Work out the finished part from the listing and answer in its coordinate system (mm). Face numbers are marked on the shaded views. A direction names the side the tool comes from. Coordinates: 2 decimals unless noted, no trailing zeros. Loops run counter-clockwise (first coordinate to the right, second up) from the corner with the lowest first, then second, coordinate; pieces in that order, holes last. Notation, with made-up numbers: (10.25, 87) - (64.25, 87) arc R24 cw to (64.25, 103) - close; hole circle Ø9 at (45, 13). An arc over 180 degrees is marked (long way). Write each question's results on one line, items separated by ' | '. Start each with the question number.
1. A cutting plane is placed at B-B on z = 0. Determine the outline of the cut face in (x, y), then the cut area to 3 significant figures.
2. Which of the six approach directions +Z, -Z, +X, -X, +Y, -Y give full straight-line access (tool end or side, diameter ignored) to the marked faces 5, 6, 7, 8 and 9?
3. Each of these flat-tipped pins is pushed along its axis until it touches: P1, Ø0.8, axis at x = 1, z = -18.5, coming from the -Y side; P2, Ø2.5, axis at x = -4, y = -10.5, coming from the -Z side; P3, Ø1.2, axis at x = -4.5, y = 1, coming from the +Z side. Where does it stop, or does it pass through?
4. A cutting plane is placed at C-C on z = -9.5. Determine the outline of the cut face in (x, y), then the cut area to 3 significant figures.
5. A cutting plane is placed at D-D on y = 2. Determine the outline of the cut face in (x, z), then the cut area to 3 significant figures.
6. Find the intervals of material crossed by line 1 along Z through (x, y) = (0, 3.4); line 2 along Y through (x, z) = (2.5, -9); line 3 along X through (y, z) = (-15.9, 0), in increasing order. Write a range as [from, to].
7. A cutting plane is placed at A-A on x = 0. Determine the outline of the cut face in (y, z), then the cut area to 3 significant figures.
8. Determine the mould class of the marked faces 1, 2, 3 and 4 for opening direction Z: released by +Z, released by -Z, zero draft, split by the parting line, or undercut.
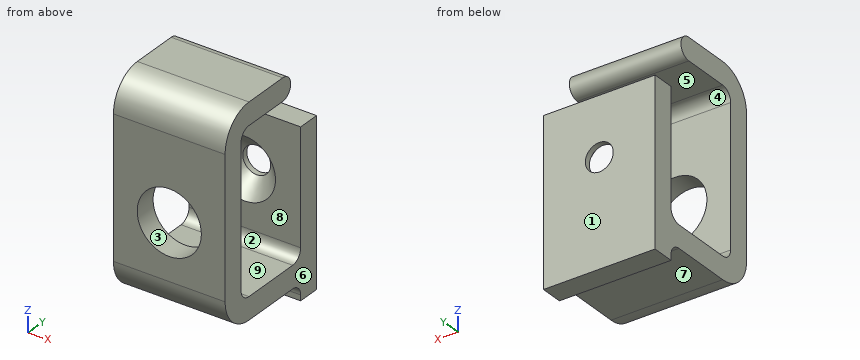
from build123d import *

# Parameters (mm, degrees)
PAD_DEPTH        = 10
HOLE_D           = 5
HOLE_CSINK_D     = 11
HOLE_CSINK_ANGLE = 90
SKETCH002_R      = 5.75
POCKET_DEPTH     = 19.001


with BuildPart() as part:
    # Sketch → Pad (new body, symmetric)
    with BuildSketch(Plane.YZ):
        with BuildLine():
            Line((0, -10), (0, 10.5))
            Line((0, 10.5), (4, 10.5))
            Line((4, 10.5), (4, -19))
            Line((4, -19), (0, -19))
            Line((0, -19), (0, -18))
            ThreePointArc((0, -18), (-0.585786, -16.585786), (-2, -16))
            Line((-2, -16), (-13, -16))
            ThreePointArc((-19, -10), (-17.242641, -14.242641), (-13, -16))
            Line((-19, -10), (-19, 15))
            ThreePointArc((-13, 21), (-17.242641, 19.242641), (-19, 15))
            Line((-13, 21), (-4.5, 21))
            ThreePointArc((-4.5, 17), (-2.5, 19), (-4.5, 21))
            Line((-13, 17), (-4.5, 17))
            ThreePointArc((-13, 17), (-14.414214, 16.414214), (-15, 15))
            Line((-15, -10), (-15, 15))
            ThreePointArc((-15, -10), (-14.414214, -11.414214), (-13, -12))
            Line((-2, -12), (-13, -12))
            ThreePointArc((-2, -12), (-0.585786, -11.414214), (0, -10))
        make_face()
    extrude(amount=PAD_DEPTH, both=True)

    # Hole (through all)
    with Locations(Plane.XZ):
        with Locations((0, 0)):
            CounterSinkHole(HOLE_D / 2, HOLE_CSINK_D / 2, counter_sink_angle=HOLE_CSINK_ANGLE)

    # Sketch002 → Pocket (cut, through all)
    with BuildSketch(Plane.XZ):
        Circle(SKETCH002_R)
    extrude(amount=POCKET_DEPTH, mode=Mode.SUBTRACT)


solid = part.part
Values:
1) outline: (-10, -19) - (-5.75, -19) - (-5.75, -15) - (-10, -15) - close; (-10, 0) - (-5.5, 0) - (-2.5, 3) - (-2.5, 4) - (-10, 4) - close; (2.5, 3) - (5.5, 0) - (10, 0) - (10, 4) - (2.5, 4) - close; (5.75, -19) - (10, -19) - (10, -15) - (5.75, -15) - close | area: 85.0 mm^2
2) face 5: +X, -X, +Y | face 6: +Z, -Z, +X, +Y, -Y | face 7: -Z, +X, -X, -Y | face 8: +Z, +X, -X | face 9: +X, -X
3) P1: y = 0 | P2: z = -16 | P3: z = 10.5
4) outline: (-10, -19) - (10, -19) - (10, -15) - (-10, -15) - close; (-10, 0) - (10, 0) - (10, 4) - (-10, 4) - close | area: 160 mm^2
5) outline: (-10, -19) - (10, -19) - (10, 10.5) - (-10, 10.5) - close; hole circle Ø7 at (0, 0) | area: 552 mm^2
6) line 1: [-19, -2.5], [2.5, 10.5] | line 2: [-19, -15], [0, 4] | line 3: [-10, -5.75], [5.75, 10]
7) outline: (-19, -10) arc R6 ccw to (-13, -16) - (-2, -16) arc R2 cw to (0, -18) - (0, -19) - (4, -19) - (4, -2.5) - (3, -2.5) - (0, -5.5) - (0, -10) arc R2 cw to (-2, -12) - (-13, -12) arc R2 cw to (-15, -10) - (-15, -5.75) - (-19, -5.75) - close; (-19, 5.75) - (-15, 5.75) - (-15, 15) arc R2 cw to (-13, 17) - (-4.5, 17) arc R2 ccw to (-4.5, 21) - (-13, 21) arc R6 ccw to (-19, 15) - close; (0, 5.5) - (3, 2.5) - (4, 2.5) - (4, 10.5) - (0, 10.5) - close | area: 287 mm^2
8) face 1: zero draft | face 2: released by +Z | face 3: undercut | face 4: undercut
